Read the model definition and answer for the solid it produces. Units are mm, in the model's axes. A direction names the side the tool comes from. Coordinates: 2 decimals unless noted, no trailing zeros. Order: outer loops, then holes, each group sorted by start corner. A loop starts at its lowest first (then second) coordinate and runs counter-clockwise, first axis right, second up. Notation, with made-up numbers: (73.5, -1) -> (107.5, -1) arc R28 ccw to (107.5, 34) -> close; hole circle Ø3 at (2.5, 61.25). An arc over 180 degrees is marked (long way). Answer in a Markdown table with one row per item.
Autodesk Inventor part; units mm, degrees
ref_plane "YZ Plane" through (0, 0, 0) normal (1, 0, 0) x (0, 1, 0)
ref_plane "XZ Plane" through (0, 0, 0) normal (0, 1, 0) x (-1, 0, 0)
ref_plane "XY Plane" through (0, 0, 0) normal (0, 0, 1) x (1, 0, 0)
sketch "Sketch1" plane through (0, 0, 0) normal (0, 0, 1) x (1, 0, 0)
  line L0 (0, 0) -> (3.75, 0)
  line L1 (3.75, 0) -> (3.75, -5)
  line L2 (3.75, -5) -> (11.25, -5)
  line L3 (11.25, -5) -> (11.25, 0)
  line L4 (11.25, 0) -> (15, 0)
  line L5 (15, 0) -> (15, 15)
  line L6 (15, 15) -> (20, 15)
  line L7 (20, 15) -> (20, 35)
  line L8 (20, 35) -> (15, 35)
  line L9 (15, 35) -> (15, 50)
  line L10 (15, 50) -> (11.25, 50)
  line L11 (11.25, 50) -> (11.25, 55)
  line L12 (11.25, 55) -> (3.75, 55)
  line L13 (3.75, 55) -> (3.75, 50)
  line L14 (3.75, 50) -> (0, 50)
  line L15 (0, 50) -> (0, 0)
  circle A0 centre (7.5, 35) radius 1.6
  circle A1 centre (7.5, 15) radius 1.6
  line L16 (7.5, 15) -> (7.5, 35)
  point P0 (20, 25)
  point P1 (0, 25)
  point P2 (7.5, -5)
  point P3 (7.5, 25)
  dimension "d0" = 5
  dimension "d1" = 50
  dimension "d2" = 20
  dimension "d3" = 7.5
  dimension "d4" = 15
  dimension "d5" = 3.2
  dimension "d6" = 20
extrude "Extrusion1" add sketch "Sketch1" along normal blind 6.731
equation "\"d7\" = THICKB"
equation "\"THICKA\" = 3.175"
equation "\"THICKB\" = 6.731"
equation "\"THICKC\" = 12.7"
equation "\"BALLDIA\" = 12"
equation "\"MAGDIA\" = 9.5"
equation "\"THICKPLY\" = 5"
properties part number "Frame_Lower_Vertical_Plate_B"
Q1. For faces 5 (the face through (3.75, -2, 3)), 6 (the face through (18, 35, 3)), 7 (the face through (3.75, 53, 3)), determine the directions among +Z, -Z, +X, -X, +Y, -Y from which every point of the face is accessible in a straight line to the end or side of a thin tool.
Outcome:
| item | result |
|---|---|
| face 5 | +Z, -Z, -X, -Y |
| face 6 | +Z, -Z, +X, +Y |
| face 7 | +Z, -Z, -X, +Y |
Q2. Given pin 1 (4 mm diameter, centred on x = 13.5, z = 2.5, fed in from +Y); pin 2 (1.9 mm diameter, centred on x = 3, z = 2, fed in from +Y); pin 3 (2.5 mm diameter, centred on x = 18, z = 2.5, fed in from -Y); pin 4 (3 mm diameter, centred on x = 13, z = 3.5, fed in from -Y), each flat-ended and moving along its own axis, determine where each tip first touches the part or whether it passes through.
Outcome:
| item | result |
|---|---|
| pin 1 | y = 50 |
| pin 2 | y = 55 |
| pin 3 | y = 15 |
| pin 4 | y = 0 |
Q3. Consider line 1 (Y direction, x = 7.5, z = 5.5); line 2 (Y direction, x = 7, z = 2); line 3 (Y direction, x = 17, z = 5.75). Determine where each line is inside the solid, lowest interval first.
Outcome:
| item | result |
|---|---|
| line 1 | -5 to 13.4, 16.6 to 33.4, 36.6 to 55 |
| line 2 | -5 to 13.48, 16.52 to 33.48, 36.52 to 55 |
| line 3 | 15 to 35 |
Q4. The part is cut by section C-C (y = 4). Write down the section's boundary in (x, z), then the cut area to 3 significant figures.
Outcome:
| item | result |
|---|---|
| outline | (0, 0) -> (15, 0) -> (15, 6.73) -> (0, 6.73) -> close |
| area | 101 mm² |
Q5. The part is cut by section A-A (x = 7.5). Write down the section's boundary in (y, z).
Outcome:
| item | result |
|---|---|
| outline | (-5, 0) -> (13.4, 0) -> (13.4, 6.73) -> (-5, 6.73) -> close; (16.6, 0) -> (33.4, 0) -> (33.4, 6.73) -> (16.6, 6.73) -> close; (36.6, 0) -> (55, 0) -> (55, 6.73) -> (36.6, 6.73) -> close |
Q6. The part is cut by section D-D (x = 2). Write down the section's boundary in (y, z).
Outcome:
| item | result |
|---|---|
| outline | (0, 0) -> (50, 0) -> (50, 6.73) -> (0, 6.73) -> close |
Q7. The part is cut by section B-B (z = 2.25). Write down the section's boundary in (x, y), then the cut area to 3 significant figures.
Outcome:
| item | result |
|---|---|
| outline | (0, 0) -> (3.75, 0) -> (3.75, -5) -> (11.25, -5) -> (11.25, 0) -> (15, 0) -> (15, 15) -> (20, 15) -> (20, 35) -> (15, 35) -> (15, 50) -> (11.25, 50) -> (11.25, 55) -> (3.75, 55) -> (3.75, 50) -> (0, 50) -> close; hole circle Ø3.2 at (7.5, 15); hole circle Ø3.2 at (7.5, 35) |
| area | 909 mm² |
Q8. For a pull along X with two mould halves and no side action, classify faces 1 (the face through (15, 42, 3)), 2 (the face through (6.32, 13.92, 3.32)), 3 (the face through (2, 0, 3)), 4 (the face through (8.24, 36.42, 3.32)) as pulls with the +X half, pulls with the -X half, needs draft (parallel to the pull), parting line crosses it, or undercut.
Outcome:
| item | result |
|---|---|
| face 1 | pulls with the +X half |
| face 2 | undercut |
| face 3 | needs draft |
| face 4 | undercut |
